from build123d import *

# Parameters (mm, degrees)
SKETCH_1_W        = 80
SKETCH_1_H        = 320
SKETCH_1_R        = 13
EXTRUDE_324_DEPTH = 8
CHAMFER_1_SIZE    = 4


with BuildPart() as part:
    # 草图1 → Extrude 324 (new body)
    with BuildSketch(Plane.XY):
        with Locations((40, 160)):
            Rectangle(SKETCH_1_W, SKETCH_1_H)
        with Locations((40, 280)):
            Circle(SKETCH_1_R, mode=Mode.SUBTRACT)
        with Locations((40, 200)):
            Circle(SKETCH_1_R, mode=Mode.SUBTRACT)
        with Locations((40, 120)):
            Circle(SKETCH_1_R, mode=Mode.SUBTRACT)
        with Locations((40, 40)):
            Circle(SKETCH_1_R, mode=Mode.SUBTRACT)
    extrude(amount=EXTRUDE_324_DEPTH)

    # 倒角1
    chamfer_1_edges = [part.edges().sort_by_distance(p)[0] for p in [
        (27, 40, 0),
        (27, 200, 0),
        (40, 0, 0),
        (80, 160, 0),
        (40, 320, 0),
        (0, 160, 0),
        (27, 280, 0),
        (27, 120, 0),
        (27, 40, 8),
        (27, 200, 8),
        (40, 320, 8),
        (80, 160, 8),
        (40, 0, 8),
        (0, 160, 8),
        (27, 280, 8),
        (27, 120, 8),
    ]]
    chamfer(chamfer_1_edges, length=CHAMFER_1_SIZE - 0.0001)  # a hair under: the kernel refuses the full size


solid = part.part
Geometry check sheet. Reference: the model listing, model coordinates, mm. Coordinates: 2 decimals unless noted, no trailing zeros. Order: outer loops, then holes, each group sorted by start corner. A loop starts at its lowest first (then second) coordinate and runs counter-clockwise, first axis right, second up. Notation, with made-up numbers: (57, 50) -> (80, 50) arc R14 ccw to (80, 62) -> close; hole circle Ø4 at (14.5, 45). An arc over 180 degrees is marked (long way). Use a Markdown table: item, result. Add a question column.
1. Cross-section at B-B (x = 40). Give the number of separate pieces and of enclosed holes in the cut face, and give its area (3 significant figures).
2. Go/stop test with flat-tipped pins: pin 1 Ø3 at (y, z) = (50, 6.5) entering from -X; pin 2 Ø1.5 at (x, z) = (18, 1.5) entering from -Y. Record where each tip stops, or that it passes through.
3. Cross-section at C-C (z = 5.5). Enter the section's corners in (x, y).
4. Material ranges on L1, parallel to Y at x = 40, z = 4; L2, parallel to X at y = 200, z = 4.05; L3, parallel to Y at x = 42, z = 4, recorded low to high.
5. Mould release check, pull along X, two halves, no side actions. Record for faces 1 (the face through (30.234, 208.955, 4.25)), 2 (the face through (39, 162, 8)): pulls with the +X half, pulls with the -X half, needs draft (parallel to the pull), parting line crosses it, or undercut.
Filled sheet:
| question | item | result |
|---|---|---|
| 1 | separate pieces | 5 |
| 1 | enclosed holes | 0 |
| 1 | area | 1,570 mm2 |
| 2 | pin 1 | x = 1 |
| 2 | pin 2 | y = 1.75 |
| 3 | outline | (1.5, 1.5) -> (78.5, 1.5) -> (78.5, 318.5) -> (1.5, 318.5) -> close; hole circle Ø29 at (40, 40); hole circle Ø29 at (40, 120); hole circle Ø29 at (40, 200); hole circle Ø29 at (40, 280) |
| 4 | L1 | 0 to 27, 53 to 107, 133 to 187, 213 to 267, 293 to 320 |
| 4 | L2 | 0.05 to 26.95, 53.05 to 79.95 |
| 4 | L3 | 0 to 27.15, 52.85 to 107.15, 132.85 to 187.15, 212.85 to 267.15, 292.85 to 320 |
| 5 | face 1 | undercut |
| 5 | face 2 | needs draft |
